Read the model definition and answer for the solid it produces. Units are mm, in the model's axes. Round coordinates to 2 decimals unless told otherwise and drop trailing zeros. Order: outer loops, then holes, each group sorted by start corner. A loop starts at its lowest first (then second) coordinate and runs counter-clockwise, first axis right, second up. Notation, with made-up numbers: (60.25, -35) -> (73.25, -35) arc R10 ccw to (73.25, -27) -> close; hole circle Ø8 at (-19.5, 23). An arc over 180 degrees is marked (long way). One line per item, written item: value. Start each with the question number.
1. Flat-ended cylindrical pins translate along their axes: pin 1 Ø5 at (x, z) = (-84.5, 130) entering from +Y; pin 2 Ø1.5 at (x, y) = (-5, 1) entering from +Z; pin 3 Ø0.9 at (y, z) = (1, 105.5) entering from -X; pin 4 Ø0.9 at (x, y) = (-116.5, 1) entering from +Z. Find the tip coordinate at first contact, or state that the pin passes through.
2. Section C-C (y = 1.1) is taken. Give the vertices of the cut face in (x, z).
3. Consider line 1 (Z direction, x = -18, y = 0.75); line 2 (X direction, y = 0.15, z = 109); line 3 (X direction, y = 1.1, z = 113.5). Determine where each line is inside the solid, lowest interval first.
4. Section D-D (z = 142.5) is taken. Give the vertices of the cut face in (x, y).
5. Section B-B (x = -38) is taken. Give the vertices of the cut face in (y, z).
6. Section A-A (z = 104.5) is taken. Give the vertices of the cut face in (x, y), then the cut area to 3 significant figures.
from build123d import *

# Parameters (mm, degrees)
LED_1_START         = 100
LED_1_OUTLINE_W     = 112
LED_1_OUTLINE_H     = 3
LED_1_DEPTH         = 25.5
LED_1_START_2       = 134.5
LED_1_2_OUTLINE_W   = 108.998029847
LED_1_2_OUTLINE_H   = 3
LED_1_2_DEPTH       = 15.5
LED_1_START_3       = 110
LED_1_3_OUTLINE_W   = 9
LED_1_3_OUTLINE_H   = 3
LED_1_3_DEPTH       = 30
LED_1_START_4       = 140
LED_1_4_OUTLINE_W   = 3.001970153
LED_1_4_OUTLINE_H   = 3
LED_1_4_DEPTH       = 4
SKETCH_1_W          = 3
SKETCH_1_H          = 34.5
CUT_EXTRUDE_1_DEPTH = 3


# Read off the part's stored shape, not the designer's step: 基体零件-LED限位板-1
with BuildPart() as part:
    # 基体零件-LED限位板-1 outline → 基体零件-LED限位板-1 (new body)
    with BuildSketch(Plane.XY.offset(LED_1_START)):
        with Locations((-59, 1.5)):
            Rectangle(LED_1_OUTLINE_W, LED_1_OUTLINE_H)
    extrude(amount=LED_1_DEPTH)



with BuildPart() as body_2:
    # LED_-1 2 outline → LED_-1 2 (new body)
    with BuildSketch(Plane.XY.offset(LED_1_START_2)):
        with Locations((-60.500985077, 1.5)):
            Rectangle(LED_1_2_OUTLINE_W, LED_1_2_OUTLINE_H)
    extrude(amount=LED_1_2_DEPTH)


with BuildPart() as part_1:
    add(part.part)

    add(body_2.part)  # LED_-1 3 merges body 2
    # LED_-1 3 outline → LED_-1 3 (add)
    with BuildSketch(Plane.XY.offset(LED_1_START_3)):
        with Locations((-113.5, 1.5)):
            Rectangle(LED_1_3_OUTLINE_W, LED_1_3_OUTLINE_H)
        with Locations((-4.5, 1.5)):
            Rectangle(LED_1_3_OUTLINE_W, LED_1_3_OUTLINE_H)
    extrude(amount=LED_1_3_DEPTH)

    # LED_-1 4 outline → LED_-1 4 (add)
    with BuildSketch(Plane.XY.offset(LED_1_START_4)):
        with Locations((-4.500985077, 1.5)):
            Rectangle(LED_1_4_OUTLINE_W, LED_1_4_OUTLINE_H)
    extrude(amount=LED_1_4_DEPTH)

    # 草图1 → 切除-拉伸1 (cut)
    with BuildSketch(Plane(origin=(0, 3, 0), x_dir=(1, 0, 0), z_dir=(0, 1, 0))):
        with Locations((-7.5, -117.25)):
            Rectangle(SKETCH_1_W, SKETCH_1_H)
    extrude(amount=-CUT_EXTRUDE_1_DEPTH, mode=Mode.SUBTRACT)


solid = part_1.part
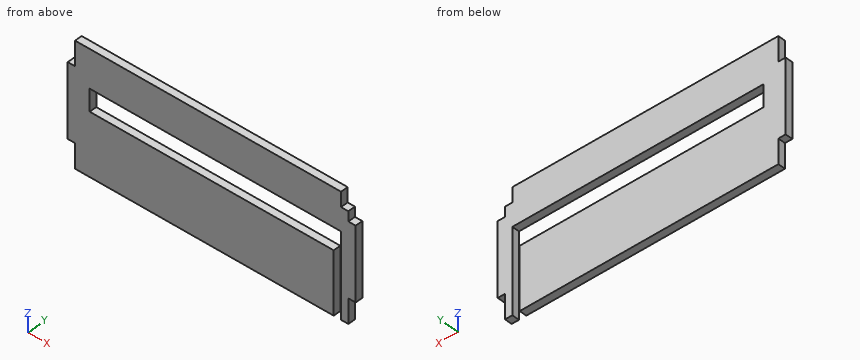
Answer:
1. pin 1: through
1. pin 2: z = 144
1. pin 3: x = -115
1. pin 4: z = 140
2. outline: (-118, 110) -> (-115, 110) -> (-115, 100) -> (-9, 100) -> (-9, 125.5) -> (-109, 125.5) -> (-109, 134.5) -> (-6, 134.5) -> (-6, 100) -> (-3, 100) -> (-3, 110) -> (0, 110) -> (0, 140) -> (-3, 140) -> (-3, 144) -> (-6, 144) -> (-6, 150) -> (-115, 150) -> (-115, 140) -> (-118, 140) -> close
3. line 1: 100 to 125.5, 134.5 to 150
3. line 2: -115 to -9, -6 to -3
3. line 3: -118 to -9, -6 to 0
4. outline: (-115, 0) -> (-3, 0) -> (-3, 3) -> (-115, 3) -> close
5. outline: (0, 100) -> (3, 100) -> (3, 125.5) -> (0, 125.5) -> close; (0, 134.5) -> (3, 134.5) -> (3, 150) -> (0, 150) -> close
6. outline: (-115, 0) -> (-9, 0) -> (-9, 3) -> (-115, 3) -> close; (-6, 0) -> (-3, 0) -> (-3, 3) -> (-6, 3) -> close
6. area: 327 mm^2
